Part model, mm, in its own coordinate system. A direction names the side the tool comes from. Give positions to 0.01 mm unless a question says otherwise; leave off trailing zeros. Write each loop counter-clockwise with the first axis right and the second up, starting at its lowest first coordinate (ties: lowest second). Pieces come first, ordered by that corner, then holes.
from build123d import *

# Parameters (mm, degrees)
F1_DEPTH  = 25.4
F3_W      = 6.35
F3_H      = 6.35
F4_W      = 6.35
F4_H      = 6.35
F5_DEPTH  = 228.6
F2_W      = 6.35
F2_H      = 6.35
F6_DEPTH  = 9.525
F8_START  = -9.525
F7_W      = 6.35
F7_H      = 6.35
F8_DEPTH  = 69.85
F9_W      = 6.35
F9_H      = 6.35
F10_DEPTH = 238.125


with BuildPart() as f1:
    # F0 (on Front) → F1 (new body)
    with BuildSketch(Plane.XZ):
        Polygon((76.2, -127), (76.2, 127), (-76.2, 127), (-76.2, -127), (-50.8, -127), (-50.8, -101.6), (-50.8, 101.6), (50.8, 101.6), (50.8, -101.6), (50.8, -127), align=None)
    extrude(amount=F1_DEPTH)

    # F3 (on face) + F4 (on face) → F5 (cut)
    with BuildSketch(Plane(origin=(0, 0, -127), x_dir=(1, 0, 0), z_dir=(0, 0, -1))):
        with Locations((-53.975, 12.7)):
            Rectangle(F3_W, F3_H)
    with BuildSketch(Plane(origin=(0, 0, -127), x_dir=(1, 0, 0), z_dir=(0, 0, -1))):
        with Locations((53.975, 12.7)):
            Rectangle(F4_W, F4_H)
    extrude(amount=-F5_DEPTH, mode=Mode.SUBTRACT)

    # F2 (on face) → F6 (cut)
    with BuildSketch(Plane(origin=(0, 0, 101.6), x_dir=(1, 0, 0), z_dir=(0, 0, -1))):
        with Locations((0, 12.7)):
            Rectangle(F2_W, F2_H)
    extrude(amount=-F6_DEPTH, mode=Mode.SUBTRACT)

    # F7 (on face) → F8 (cut)
    with BuildSketch(Plane.YZ.offset(76.2).offset(F8_START)):
        with Locations((-12.7, 114.3)):
            Rectangle(F7_W, F7_H)
    extrude(amount=-F8_DEPTH, mode=Mode.SUBTRACT)

    # F9 (on face) → F10 (cut)
    with BuildSketch(Plane(origin=(0, 0, -127), x_dir=(1, 0, 0), z_dir=(0, 0, -1))):
        with Locations((63.5, 12.7)):
            Rectangle(F9_W, F9_H)
    extrude(amount=-F10_DEPTH, mode=Mode.SUBTRACT)


solid = f1.part
1) Saw through at A-A (z = 35). Write the cut outline in (x, y) (3 decimals), and give its area (3 significant figures).
Check result:
outline: (-76.2, -25.4) - (-50.8, -25.4) - (-50.8, -15.875) - (-57.15, -15.875) - (-57.15, -9.525) - (-50.8, -9.525) - (-50.8, 0) - (-76.2, 0) - close; (50.8, -25.4) - (76.2, -25.4) - (76.2, 0) - (50.8, 0) - (50.8, -9.525) - (57.15, -9.525) - (57.15, -15.875) - (50.8, -15.875) - close; hole (60.325, -15.875) - (66.675, -15.875) - (66.675, -9.525) - (60.325, -9.525) - close
area: 1,170 mm2
2) Mould opens along Z. For faces 6 (the flat face through (32, -13, 117.475)), 7 (the flat face through (-50.8, -21, -14)), 8 (the flat face through (1, -13, 127)) say: +Z half, -Z half, draft (parallel to the pull), parting line (faces both ways), or undercut.
Check result:
face 6: undercut
face 7: draft
face 8: +Z half
3) Saw through at C-C (x = 32.5). Write the cut outline in (y, z) (3 decimals).
Check result:
outline: (-25.4, 101.6) - (0, 101.6) - (0, 127) - (-25.4, 127) - close; hole (-15.875, 111.125) - (-9.525, 111.125) - (-9.525, 117.475) - (-15.875, 117.475) - close
4) Drill centre lines: L1, parallel to X at y = -15.25, z = 83.5 (3 decimals); L2, parallel to Y at x = 61, z = -23 (3 decimals); L3, parallel to X at y = -5.5, z = -52. Where is each one in solid material? Low to high.
Check result:
L1: x = -76.2 to -57.15, 57.15 to 60.325, 66.675 to 76.2
L2: y = -25.4 to -15.875, -9.525 to 0
L3: x = -76.2 to -50.8, 50.8 to 76.2
5) Saw through at D-D (x = -7). Write the cut outline in (y, z), and give its area (3 significant figures).
Check result:
outline: (-25.4, 101.6) - (0, 101.6) - (0, 127) - (-25.4, 127) - close
area: 645 mm2
6) 3-axis set-ups, long thin cutter, end or side, ignore diameter. For faces 1 (the flat face through (-52, 0, 30)), 2 (the flat face through (69, -13, -127)), 3 (the flat face through (63, -9.525, 31)), 4 (the flat face through (50.8, -5, -11)), 5 (the flat face through (3.175, -13, 106)): which of +Z, -Z, +X, -X, +Y, -Y reach the whole face in a straight line?
Check result:
face 1: +Z, -Z, +X, -X, +Y
face 2: -Z, +X, -X, +Y, -Y
face 3: none
face 4: -Z, +Y, -Y
face 5: -Z
7) Flat gauge pin, fed straight in: P1, Ø7.5, axis at x = 13, y = -15, coming from the -Z side. Where does the tip first touch, or does it go through?
Check result:
P1: stops at z = 101.6
8) Saw through at B-B (y = -12.5). Write the cut outline in (x, z) (3 decimals).
Check result:
outline: (-76.2, -127) - (-57.15, -127) - (-57.15, 101.6) - (-3.175, 101.6) - (-3.175, 117.475) - (66.675, 117.475) - (66.675, -127) - (76.2, -127) - (76.2, 127) - (-76.2, 127) - close; (3.175, 101.6) - (57.15, 101.6) - (57.15, -127) - (60.325, -127) - (60.325, 111.125) - (3.175, 111.125) - close
